from build123d import *

# Parameters (mm, degrees)
F0_W     = 44.126308
F0_H     = 20.30415
F1_DEPTH = 5
F2_W     = 3.175
F2_H     = 20.30415
F3_DEPTH = 5
F4_R     = 1.9
F4_R_2   = 1.85
F5_DEPTH = 10.001


with BuildPart() as f1:
    # F0 (on Top) → F1 (new body)
    with BuildSketch(Plane.XY):
        with Locations((-22.84455, -40.602903)):
            Rectangle(F0_W, F0_H)
    extrude(amount=-F1_DEPTH)

    # F2 (on face) → F3 (join)
    with BuildSketch(Plane.XY):
        with Locations((-7.086134, -40.602903)):
            Rectangle(F2_W, F2_H)
        with Locations((-13.944134, -40.602903)):
            Rectangle(F2_W, F2_H)
        with Locations((-20.040134, -40.602903)):
            Rectangle(F2_W, F2_H)
        with Locations((-26.644134, -40.602903)):
            Rectangle(F2_W, F2_H)
        with Locations((-32.994134, -40.602903)):
            Rectangle(F2_W, F2_H)
    extrude(amount=F3_DEPTH)

    # F4 (on face) → F5 (cut, through all)
    with BuildSketch(Plane(origin=(0, 0, -5), x_dir=(1, 0, 0), z_dir=(0, 0, -1))):
        with Locations((-40.255573, 45.675743)):
            Circle(F4_R)
        with Locations((-40.718783, 36.96854)):
            Circle(F4_R_2)
    extrude(amount=-F5_DEPTH, mode=Mode.SUBTRACT)


solid = f1.part
Design review of the part built by this model. Coordinates are the model's own, in mm. A direction names the side the tool comes from. Give positions to 0.01 mm unless a question says otherwise; leave off trailing zeros. Order: outer loops, then holes, each group sorted by start corner. A loop starts at its lowest first (then second) coordinate and runs counter-clockwise, first axis right, second up.
1. Add section B-B, the plane y = -38. State the section outline as (x, z) points, then the cut area to 3 significant figures.
Solution:
outline: (-44.91, -5) - (-42.25, -5) - (-42.25, 0) - (-44.91, 0) - close; (-39.18, -5) - (-0.78, -5) - (-0.78, 0) - (-5.5, 0) - (-5.5, 5) - (-8.67, 5) - (-8.67, 0) - (-12.36, 0) - (-12.36, 5) - (-15.53, 5) - (-15.53, 0) - (-18.45, 0) - (-18.45, 5) - (-21.63, 5) - (-21.63, 0) - (-25.06, 0) - (-25.06, 5) - (-28.23, 5) - (-28.23, 0) - (-31.41, 0) - (-31.41, 5) - (-34.58, 5) - (-34.58, 0) - (-39.18, 0) - close
area: 285 mm2
2. Add section A-A, the plane z = 3.25. State the section outline as (x, y) points, then the cut area to 3 significant figures.
Solution:
outline: (-34.58, -50.75) - (-31.41, -50.75) - (-31.41, -30.45) - (-34.58, -30.45) - close; (-28.23, -50.75) - (-25.06, -50.75) - (-25.06, -30.45) - (-28.23, -30.45) - close; (-21.63, -50.75) - (-18.45, -50.75) - (-18.45, -30.45) - (-21.63, -30.45) - close; (-15.53, -50.75) - (-12.36, -50.75) - (-12.36, -30.45) - (-15.53, -30.45) - close; (-8.67, -50.75) - (-5.5, -50.75) - (-5.5, -30.45) - (-8.67, -30.45) - close
area: 322 mm2
3. For pin 1 Ø5.5 at (y, z) = (-43, 3) entering from -X; pin 2 Ø4 at (y, z) = (-42, 2.5) entering from +X; pin 3 Ø11.5 at (x, y) = (-40.5, -39.5) entering from +Z, all flat-tipped, find the tip position at first contact; note any pin that passes through.
Solution:
pin 1: stops at x = -34.58
pin 2: stops at x = -5.5
pin 3: stops at z = 0
4. Mouldability with a two-part tool opening along X and no side actions: class faces 4 (the flat face through (-11, -40, 0)), 5 (the flat face through (-34.582, -41, 2)), 6 (the flat face through (-7, -40, 5)) as +X half, -X half, draft (parallel to the pull), parting line (faces both ways), or undercut.
Solution:
face 4: undercut
face 5: -X half
face 6: draft
5. To check wall thickness, follow L1, parallel to X at y = -46.25, z = 3.25; L2, parallel to Z at x = -16.5, y = -37.5; L3, parallel to X at y = -45, z = -2.75. State the ranges of each line that lie inside material, in increasing order.
Solution:
L1: x = -34.58 to -31.41, -28.23 to -25.06, -21.63 to -18.45, -15.53 to -12.36, -8.67 to -5.5
L2: z = -5 to 0
L3: x = -44.91 to -42.03, -38.48 to -0.78
6. Add section C-C, the plane x = -41. State the section outline as (y, z) points.
Solution:
outline: (-50.75, -5) - (-47.42, -5) - (-47.42, 0) - (-50.75, 0) - close; (-43.93, -5) - (-38.8, -5) - (-38.8, 0) - (-43.93, 0) - close; (-35.14, -5) - (-30.45, -5) - (-30.45, 0) - (-35.14, 0) - close
7. Add section D-D, the plane y = -34.5. State the section outline as (x, z) points.
Solution:
outline: (-44.91, -5) - (-0.78, -5) - (-0.78, 0) - (-5.5, 0) - (-5.5, 5) - (-8.67, 5) - (-8.67, 0) - (-12.36, 0) - (-12.36, 5) - (-15.53, 5) - (-15.53, 0) - (-18.45, 0) - (-18.45, 5) - (-21.63, 5) - (-21.63, 0) - (-25.06, 0) - (-25.06, 5) - (-28.23, 5) - (-28.23, 0) - (-31.41, 0) - (-31.41, 5) - (-34.58, 5) - (-34.58, 0) - (-44.91, 0) - close
8. Tool access review of faces 1 (the flat face through (-23, -40, 0)), 2 (the flat face through (-40, -40, 0)), 3 (the flat face through (-3, -40, 0)): name each direction out of +Z, -Z, +X, -X, +Y, -Y from which nothing blocks a thin tool from reaching the whole face with its end or side.
Solution:
face 1: +Z, +Y, -Y
face 2: +Z, -X, +Y, -Y
face 3: +Z, +X, +Y, -Y
